Autodesk Inventor part; units mm, degrees
ref_plane "YZ Plane" through (0, 0, 0) normal (1, 0, 0) x (0, 1, 0)
ref_plane "XZ Plane" through (0, 0, 0) normal (0, 1, 0) x (-1, 0, 0)
ref_plane "XY Plane" through (0, 0, 0) normal (0, 0, 1) x (1, 0, 0)
sketch "スケッチ1" plane through (0, 0, 0) normal (0, 0, 1) x (1, 0, 0)
  circle A0 centre (0, 0) radius 21.25
  circle A1 centre (0, 0) radius 36.55
  line L0 (0, 0) -> (-28.1908, 10.2606) construction
  line L1 (0, 0) -> (28.1908, 10.2606) construction
  line L2 (-39.5959, 0) -> (43.1917, 0) construction
  line L3 (0, 0) -> (0, 30) construction
  circle A2 centre (-28.1908, 10.2606) radius 2.55
  circle A3 centre (0, 30) radius 2.55
  circle A4 centre (28.1908, 10.2606) radius 2.55
  dimension "d0" = 73.1
  dimension "d1" = 42.5
  dimension "d2" = 30
  dimension "d3" = 30
  dimension "d4" = 20
  dimension "d5" = 20
  dimension "d6" = 30
  dimension "d7" = 5.1
  dimension "d8" = 5.1
  dimension "d9" = 5.1
extrude "押し出し1" add sketch "スケッチ1" along normal blind 5
sketch "スケッチ2" plane through (0, 0, 5) normal (0, 0, 1) x (1, 0, 0)
  line L0 (0, 0) -> (0, -80) construction
  circle A0 centre (0, -80) radius 52.5
  dimension "d12" = 80
  dimension "d16" = 105
extrude "押し出し2" cut sketch "スケッチ2" against normal blind 10
sketch "スケッチ3" plane through (0, 0, 5) normal (0, 0, 1) x (1, 0, 0)
  arc A0 (19.1643, -31.1228) -> (-19.1643, -31.1228) centre (0, 0) ccw
  line L0 (31.4805, -18.571) -> (8.7644, -29.8131)
  line L1 (8.7644, -29.8131) -> (11.2377, -39.3237)
  line L2 (11.2377, -39.3237) -> (35.6526, -33.4076)
  line L3 (35.6526, -33.4076) -> (31.4805, -18.571)
extrude "押し出し3" cut sketch "スケッチ3" against normal blind 10
properties part number "円 42.5mm" material "アルミニウム 6061"
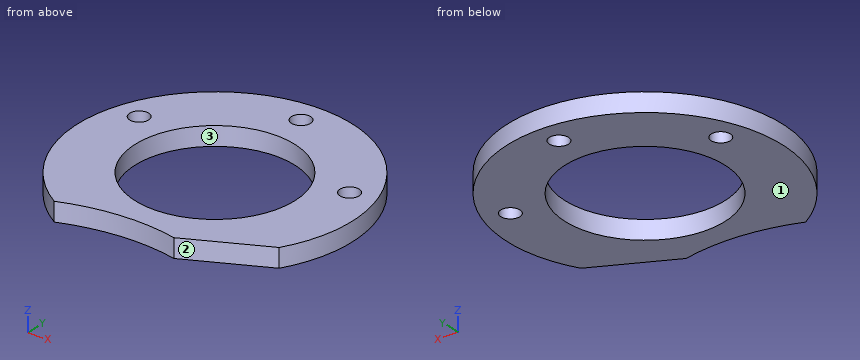
Design review of the part built by this model. Coordinates are the model's own, in mm. Face numbers are marked on the shaded views. Give positions to 0.01 mm unless a question says otherwise; leave off trailing zeros. Loops run counter-clockwise (first coordinate to the right, second up) from the corner with the lowest first, then second, coordinate; pieces in that order, holes last. Notation, with made-up numbers: M 13.25,-35 L 43.25,-35 A26 ccw 43.25,-17 Z; hole C -39.5,68 d5. An arc over 180 degrees is marked long. One line per question, with ' | ' between items. Start each with the question number.
1. To check wall thickness, follow L1, parallel to Y at x = 0, z = 1.3; L2, parallel to X at y = 8, z = 3.3; L3, parallel to X at y = 11.5, z = 4.25. State the ranges of each line that lie inside material, in increasing order.
2. Add section A-A (y = 0). Write out the cut boundary in (x, z), plus the area to 3 significant figures.
3. Insertion check: P1, Ø1, axis at y = -4.5, z = 3.5, coming from the +X side; P2, Ø4.5, axis at x = -28.19, y = 10.26, coming from the -Z side; P3, Ø3, axis at x = 15, z = 1, coming from the -Y side. Each pin has a flat end and moves straight along its axis. Give the tip position at first contact, or say it passes through.
4. Add section B-B (x = 0). Write out the cut boundary in (y, z), plus the area to 4 significant figures.
5. The part is to be moulded in two halves that separate along X. For the marked faces 1, 2 and 3, say which applies: released by +X, released by -X, zero draft, split by the parting line, or undercut.
6. Add section D-D (y = 30). Write out the cut boundary in (x, z).
7. Add section C-C (z = 3.25). Write out the cut boundary in (x, y).
Worked out:
1) L1: y = -27.5 to -21.25, 21.25 to 27.45, 32.55 to 36.55 | L2: x = -35.66 to -29.37, -27.01 to -19.69, 19.69 to 27.01, 29.37 to 35.66 | L3: x = -34.69 to -30.42, -25.96 to -17.87, 17.87 to 25.96, 30.42 to 34.69
2) outline: M -36.55,0 L -21.25,0 L -21.25,5 L -36.55,5 Z; M 21.25,0 L 36.55,0 L 36.55,5 L 21.25,5 Z | area: 153 mm²
3) P1: stops at x = 36.33 | P2: passes through | P3: stops at y = -27.47
4) outline: M -27.5,0 L -21.25,0 L -21.25,5 L -27.5,5 Z; M 21.25,0 L 27.45,0 L 27.45,5 L 21.25,5 Z; M 32.55,0 L 36.55,0 L 36.55,5 L 32.55,5 Z | area: 82.25 mm²
5) face 1: zero draft | face 2: released by +X | face 3: undercut
6) outline: M -20.88,0 L -2.55,0 L -2.55,5 L -20.88,5 Z; M 2.55,0 L 20.88,0 L 20.88,5 L 2.55,5 Z
7) outline: M -19.16,-31.12 A52.5 cw 11.06,-28.68 L 31.48,-18.57 A36.55 ccw long Z; hole C -28.19,10.26 d5.1; hole C 0,0 d42.5; hole C 0,30 d5.1; hole C 28.19,10.26 d5.1
